```python
from build123d import *

# Parameters (mm, degrees)
SKETCH1_R           = 11
BOSS_EXTRUDE1_DEPTH = 10
SKETCH2_R           = 3
CUT_EXTRUDE1_DEPTH  = 20
SKETCH5_R           = 10
CUT_EXTRUDE3_DEPTH  = 5


with BuildPart() as part:
    # Sketch1 → Boss-Extrude1 (new body)
    with BuildSketch(Plane(origin=(0, 0, 0), x_dir=(1, 0, 0), z_dir=(0, 1, 0))):
        with Locations(Location((0, 0, 0), (0, 0, 270))):
            Circle(SKETCH1_R)
    extrude(amount=BOSS_EXTRUDE1_DEPTH)

    # Sketch2 → Cut-Extrude1 (cut)
    with BuildSketch(Plane(origin=(0, 0, 0), x_dir=(1, 0, 0), z_dir=(0, 1, 0))):
        with Locations(Location((0, 0, 0), (0, 0, 270))):
            Circle(SKETCH2_R)
    extrude(amount=CUT_EXTRUDE1_DEPTH, mode=Mode.SUBTRACT)

    # Sketch5 → Cut-Extrude3 (cut)
    with BuildSketch(Plane(origin=(0, 10, 0), x_dir=(1, 0, 0), z_dir=(0, 1, 0))):
        with Locations(Location((0, 0, 0), (0, 0, 270))):
            Circle(SKETCH5_R)
    extrude(amount=-CUT_EXTRUDE3_DEPTH, mode=Mode.SUBTRACT)


solid = part.part
```
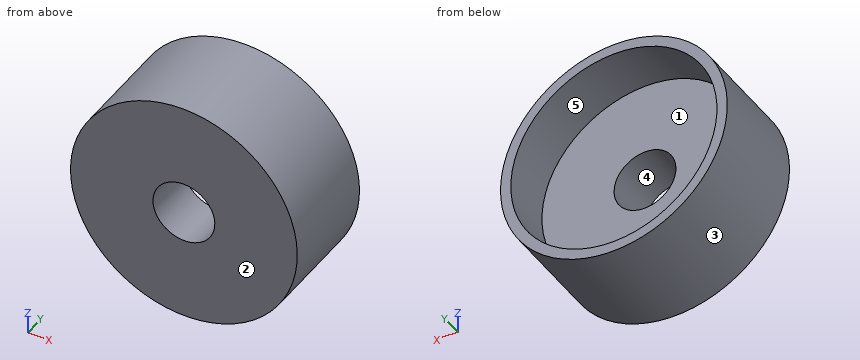
Design review of the part built by this model. Coordinates are the model's own, in mm. Face numbers are marked on the shaded views. A direction names the side the tool comes from. Round coordinates to 2 decimals unless told otherwise and drop trailing zeros. Write each loop counter-clockwise with the first axis right and the second up, starting at its lowest first coordinate (ties: lowest second). Pieces come first, ordered by that corner, then holes. Notation, with made-up numbers: (-1.75, -7) -> (2.25, -7) arc R19 ccw to (2.25, 9) -> close; hole circle Ø8 at (45, 5). An arc over 180 degrees is marked (long way). Answer in a Markdown table with one row per item.
Q1. Draft analysis for pull direction X (two halves, no side actions). For the marked faces 1, 2 and 3, state which applies: +X half, -X half, draft (parallel to the pull), parting line (faces both ways), or undercut.
The answers:
| item | result |
|---|---|
| face 1 | undercut |
| face 2 | draft |
| face 3 | parting line |
Q2. Clearance check with flat-ended pins moving along their axes: pin 1 Ø3 at (y, z) = (5.5, 4) entering from -X; pin 2 Ø3 at (x, z) = (-4, 3) entering from -Y; pin 3 Ø1 at (y, z) = (4.5, 5.5) entering from +X; pin 4 Ø5 at (y, z) = (4.5, 6.5) entering from +X. State where each tip first meets the part, or that it passes through.
The answers:
| item | result |
|---|---|
| pin 1 | x = -10.71 |
| pin 2 | y = 0 |
| pin 3 | x = 9.8 |
| pin 4 | x = 10.25 |
Q3. To check wall thickness, follow L1, parallel to X at y = 1.45, z = 0; L2, parallel to Z at x = -0.25, y = 8.5. State the ranges of each line that lie inside material, in increasing order. Write a range as [from, to].
The answers:
| item | result |
|---|---|
| L1 | [-11, -3], [3, 11] |
| L2 | [-11, -10], [10, 11] |
Q4. Take a section at B-B, the plane x = 2. State the section outline as (y, z) points.
The answers:
| item | result |
|---|---|
| outline | (0, -10.82) -> (10, -10.82) -> (10, -9.8) -> (5, -9.8) -> (5, -2.24) -> (0, -2.24) -> close; (0, 2.24) -> (5, 2.24) -> (5, 9.8) -> (10, 9.8) -> (10, 10.82) -> (0, 10.82) -> close |
Q5. Take a section at A-A, the plane z = 0. State the section outline as (x, y) points, then the cut area to 3 significant figures.
The answers:
| item | result |
|---|---|
| outline | (-11, 0) -> (-3, 0) -> (-3, 5) -> (-10, 5) -> (-10, 10) -> (-11, 10) -> close; (3, 0) -> (11, 0) -> (11, 10) -> (10, 10) -> (10, 5) -> (3, 5) -> close |
| area | 90.0 mm² |
Q6. Take a section at D-D, the plane z = 5.75. State the section outline as (x, y) points.
The answers:
| item | result |
|---|---|
| outline | (-9.38, 0) -> (9.38, 0) -> (9.38, 10) -> (8.18, 10) -> (8.18, 5) -> (-8.18, 5) -> (-8.18, 10) -> (-9.38, 10) -> close |
Q7. Take a section at C-C, the plane y = 0.5. State the section outline as (x, z) points, then the cut area to 3 significant figures.
The answers:
| item | result |
|---|---|
| outline | circle Ø22 at (0, 0); hole circle Ø6 at (0, 0) |
| area | 352 mm² |
Q8. For the marked faces 4 and 5, list the 3-axis set-ups (+Z, -Z, +X, -X, +Y, -Y) from which the entire face can be reached by the end or side of a thin tool; tool diameter is ignored.
The answers:
| item | result |
|---|---|
| face 4 | +Y, -Y |
| face 5 | +Y |
